Could you check a few things on this model? Use its own coordinates, in mm. A direction names the side the tool comes from. Coordinates: 2 decimals unless noted, no trailing zeros. Order: outer loops, then holes, each group sorted by start corner. A loop starts at its lowest first (then second) coordinate and runs counter-clockwise, first axis right, second up. Notation, with made-up numbers: (-31, 22) - (4, 22) arc R21 cw to (4, 45) - close; hole circle Ø5 at (35, 54.25). An arc over 180 degrees is marked (long way). One line per item, written item: value.
from build123d import *

# Parameters (mm, degrees)
RESSALTO_EXTRUS_O1_DEPTH      = 3
RESSALTO_EXTRUS_O1_DEPTH_BACK = 0.6
ESBO_O1_W                     = 119
ESBO_O1_H                     = 62
ESBO_O1_R                     = 7.5
RESSALTO_EXTRUS_O2_DEPTH      = 9
CORTE_EXTRUS_O1_START         = -2
CORTE_EXTRUS_O1_DEPTH         = 133.772994327
ESBO_O4_R                     = 3
CORTE_EXTRUS_O2_DEPTH         = 28
CORTE_EXTRUS_O3_START         = -3
ESBO_O4_4_R                   = 6.25
ESBO_O4_4_R_2                 = 3
CORTE_EXTRUS_O3_DEPTH         = 25
ESBO_O6_R                     = 0.75
CORTE_EXTRUS_O5_DEPTH         = 3.6
CORTE_EXTRUS_O6_REACH         = 136.773
ESBO_O7_W                     = 10
ESBO_O7_H                     = 17
FILETE1_R                     = 4


with BuildPart() as part:
    # Esboço1 → Ressalto-extrusão1 (new, two sides: drawn at the far end of the back side and taken through both)
    with BuildSketch(Plane(origin=(0, 0, 0), x_dir=(1, 0, 0), z_dir=(0, 1, 0)).offset(-RESSALTO_EXTRUS_O1_DEPTH_BACK)):
        with Locations((59.5, 31)):
            Rectangle(ESBO_O1_W, ESBO_O1_H)
        with Locations(Location((20, 52, 0), (0, 0, 270))):
            Circle(ESBO_O1_R, mode=Mode.SUBTRACT)
        with Locations(Location((20, 12, 0), (0, 0, 270))):
            Circle(ESBO_O1_R, mode=Mode.SUBTRACT)
    extrude(amount=RESSALTO_EXTRUS_O1_DEPTH + RESSALTO_EXTRUS_O1_DEPTH_BACK)

    # Esboço2 → Ressalto-extrusão2 (add)
    with BuildSketch(Plane(origin=(0, 3, 0), x_dir=(1, 0, 0), z_dir=(0, 1, 0))):
        Polygon((47, 2), (115, 2), (115, 60), (47, 60), (47, 40), (0, 40), (0, 22), (47, 22), align=None)
    extrude(amount=RESSALTO_EXTRUS_O2_DEPTH)

    # Esboço3 → Corte-extrusão1 (cut, through all)
    with BuildSketch(Plane(origin=(0, 12, 0), x_dir=(1, 0, 0), z_dir=(0, 1, 0)).offset(CORTE_EXTRUS_O1_START)):
        Polygon((49, 58), (113, 58), (113, 4), (49, 4), (49, 25), (3, 25), (3, 37), (49, 37), align=None)
    extrude(amount=-CORTE_EXTRUS_O1_DEPTH, mode=Mode.SUBTRACT)

    # Esboço4 → Corte-extrusão2 (cut)
    with BuildSketch(Plane.ZY):
        with Locations((-31, 5.9)):
            Circle(ESBO_O4_R)
    extrude(amount=-CORTE_EXTRUS_O2_DEPTH, mode=Mode.SUBTRACT)

    # Esboço4<4> → Corte-extrusão3 (cut)
    with BuildSketch(Plane.ZY.offset(CORTE_EXTRUS_O3_START)):
        with Locations((-31, 5.9)):
            Circle(ESBO_O4_4_R)
        with Locations((-31, 5.9)):
            Circle(ESBO_O4_4_R_2, mode=Mode.SUBTRACT)
    extrude(amount=-CORTE_EXTRUS_O3_DEPTH, mode=Mode.SUBTRACT)

    # Esboço6 → Corte-extrusão5 (cut)
    with BuildSketch(Plane.XZ.offset(0.6)):
        with Locations((114.2, 0)):
            Circle(ESBO_O6_R)
        with Locations((114.2, -62)):
            Circle(ESBO_O6_R)
    extrude(amount=-CORTE_EXTRUS_O5_DEPTH, mode=Mode.SUBTRACT)

    # Corte-extrusão6: up to this face of the body (flat: up to its plane)
    corte_extrus_o6_end = Plane(part.part.faces().sort_by_distance((71.642099046, 12, -31))[0])
    # Esboço7 → Corte-extrusão6 (cut, up to the picked face)
    with BuildSketch(Plane(origin=(0, -0.6, 0), x_dir=(-1, 0, 0), z_dir=(0, -1, 0)), mode=Mode.PRIVATE) as corte_extrus_o6_sk1:
        with Locations((-114, 49.5)):
            Rectangle(ESBO_O7_W, ESBO_O7_H)
    corte_extrus_o6_tool1 = split(extrude(corte_extrus_o6_sk1.sketch, amount=-CORTE_EXTRUS_O6_REACH, mode=Mode.PRIVATE), bisect_by=corte_extrus_o6_end, keep=Keep.BOTH, mode=Mode.PRIVATE)
    add(corte_extrus_o6_tool1.solids().sort_by(Axis((114, -0.6, -49.5), (0, 1, 0)))[0], mode=Mode.SUBTRACT)

    # Filete1
    # the kernel refuses this fillet: 4 mm, written as the material it takes off along each edge
    with BuildSketch(Plane(origin=(0, 12, -50), x_dir=(1, 0, 0), z_dir=(0, 0, 1))) as filete1_piece_1:
        with BuildLine():
            CenterArc((FILETE1_R, -FILETE1_R), FILETE1_R, 90, 90)
            Line((0, -FILETE1_R), (0, 0))
            Line((0, 0), (FILETE1_R, 0))
        make_face()
    extrude(amount=38, mode=Mode.SUBTRACT)


solid = part.part
Item 1: For faces 4 (the face through (26, 4, -25)), 5 (the face through (47, 7, -50)), 6 (the face through (84, 4, -58)), 7 (the face through (15.32, 5.88, -24.75)), which set-ups out of +Z, -Z, +X, -X, +Y, -Y let a thin tool reach every point of the face, with its end or its side?
Conclusion:
face 4: -Y
face 5: -Z, -X, +Y
face 6: +X, -Y
face 7: none
Item 2: Thinking about a two-plate mould opening in Z: for faces 1 (the face through (81, 5, -4)), 2 (the face through (47, 7, -12)), 3 (the face through (81, 7, -60)), which applies, pulls with the +Z half, pulls with the -Z half, needs draft (parallel to the pull), parting line crosses it, or undercut?
Conclusion:
face 1: undercut
face 2: needs draft
face 3: pulls with the -Z half
Item 3: I want a section at C-C on x = 20. Please give me the cut outline in (y, z).
Conclusion:
outline: (-0.6, -62) - (3, -62) - (3, -59.5) - (-0.6, -59.5) - close; (-0.6, -44.5) - (3, -44.5) - (3, -40) - (12, -40) - (12, -32.36) arc R6.25 cw to (10, -35.72) - (10, -37) - (7.65, -37) arc R6.25 cw to (4.15, -37) - (-0.6, -37) - close; (-0.6, -25) - (4.15, -25) arc R6.25 cw to (7.65, -25) - (10, -25) - (10, -26.28) arc R6.25 cw to (12, -29.64) - (12, -22) - (3, -22) - (3, -19.5) - (-0.6, -19.5) - close; (-0.6, -4.5) - (3, -4.5) - (3, 0) - (-0.6, 0) - close
Item 4: I want a section at A-A on z = -12. Please give me the cut outline in (x, y), then the cut area to 3 significant figures.
Conclusion:
outline: (0, -0.6) - (12.5, -0.6) - (12.5, 3) - (0, 3) - close; (27.5, -0.6) - (49, -0.6) - (49, 10) - (113, 10) - (113, -0.6) - (119, -0.6) - (119, 3) - (115, 3) - (115, 12) - (47, 12) - (47, 3) - (27.5, 3) - close
area: 308 mm²
Item 5: If I drill on probe 1 along Z at (x, y) = (52, 3.5); probe 2 along X at (y, z) = (2.2, -12); probe 3 along Z at (x, y) = (70.5, 0), over which ranges is the centre line in solid material (lowest first)?
Conclusion:
probe 1: -60 to -58, -4 to -2
probe 2: 0 to 12.5, 27.5 to 49, 113 to 119
probe 3: -62 to -58, -4 to 0
Item 6: I want a section at D-D on y = 0.5. Please give me the cut outline in (x, z).
Conclusion:
outline: (0, -62) - (113.45, -62) arc R0.75 cw to (114.95, -62) - (119, -62) - (119, -58) - (49, -58) - (49, -37) - (3, -37) - (3, -25) - (49, -25) - (49, -4) - (113, -4) - (113, -41) - (119, -41) - (119, 0) - (114.95, 0) arc R0.75 cw to (113.45, 0) - (0, 0) - close; hole circle Ø15 at (20, -52); hole circle Ø15 at (20, -12)
Item 7: I want a section at B-B on y = 5.9. Please give me the cut outline in (x, z), then the cut area to 4 significant figures.
Conclusion:
outline: (0, -40) - (47, -40) - (47, -60) - (115, -60) - (115, -58) - (49, -58) - (49, -37) - (28, -37) - (28, -37.25) - (3, -37.25) - (3, -34) - (0, -34) - close; (0, -28) - (3, -28) - (3, -24.75) - (28, -24.75) - (28, -25) - (49, -25) - (49, -4) - (113, -4) - (113, -41) - (115, -41) - (115, -2) - (47, -2) - (47, -22) - (0, -22) - close
area: 717.5 mm²
Item 8: I'm going to push flat-ended pins straight in: pin 1 Ø1.5 at (y, z) = (5.5, -19.5) entering from -X; pin 2 Ø3 at (x, y) = (15.5, 5.5) entering from +Z; pin 3 Ø6 at (y, z) = (10.5, -16) entering from +X; pin 4 Ø1.5 at (x, z) = (13.5, -11.5) entering from -Y. Where does each tip first touch, or does it pass through?
Conclusion:
pin 1: x = 47
pin 2: z = -22
pin 3: x = 115
pin 4: through
